```python
from build123d import *

# Parameters (mm, degrees)
SKETCH1_R           = 45
BOSS_EXTRUDE2_DEPTH = 2.5
BOSS_EXTRUDE4_START = -2.5
BOSS_EXTRUDE4_DEPTH = 2.5
CIRPATTERN1_COUNT   = 6
CUT_EXTRUDE2_DEPTH  = 2.5
SKETCH6_R           = 1.5
CUT_EXTRUDE3_DEPTH  = 5
SKETCH7_R           = 1.5875
CUT_EXTRUDE4_DEPTH  = 2.5


with BuildPart() as part:
    # Sketch1 → Boss-Extrude2 (new body)
    with BuildSketch(Plane(origin=(0, 0, 0), x_dir=(1, 0, 0), z_dir=(0, 1, 0))):
        with Locations(Location((0, 0, 0), (0, 0, 270))):
            Circle(SKETCH1_R)
    extrude(amount=BOSS_EXTRUDE2_DEPTH)

    # Sketch2 → Boss-Extrude4 (add)
    with BuildSketch(Plane(origin=(0, 2.5, 0), x_dir=(1, 0, 0), z_dir=(0, 1, 0)).offset(BOSS_EXTRUDE4_START)):
        with BuildLine():
            ThreePointArc((-42.23454554, 15.532004475), (-45, 0), (-42.23454554, -15.532004475))
            add(Edge.make_bspline(
                [(-50.212380227, -7.942360629), (-45.3159648, -11.95963121), (-42.656686571, -14.489512492), (-42.23454554, -15.532004475)],
                knots=[0.089311832, 0.089311832, 0.089311832, 0.089311832, 1, 1, 1, 1], degree=3))
            ThreePointArc((-50.212380227, -7.942360629), (-54.5, 0), (-50.212380227, 7.942360629))
            add(Edge.make_bspline(
                [(-50.212380227, 7.942360629), (-45.3159648, 11.95963121), (-42.656686571, 14.489512492), (-42.23454554, 15.532004475)],
                knots=[0.089311832, 0.089311832, 0.089311832, 0.089311832, 1, 1, 1, 1], degree=3))
        make_face()
    boss_extrude4 = extrude(amount=BOSS_EXTRUDE4_DEPTH)

    # CirPattern1: Boss-Extrude4 ×6 about axis
    cirpattern1_axis = Axis((0, 2.5, 0), (0, 1, 0))
    for i in range(1, CIRPATTERN1_COUNT):
        add(boss_extrude4.rotate(cirpattern1_axis, i * 360 / CIRPATTERN1_COUNT))

    # Sketch5 → Cut-Extrude2 (cut)
    with BuildSketch(Plane(origin=(0, 2.5, 0), x_dir=(1, 0, 0), z_dir=(0, 1, 0))):
        with BuildLine():
            Line((-8.22468756, 44.342191593), (0, 46.65782144))
            Line((0, 46.65782144), (8.22468756, 44.342191593))
            ThreePointArc((8.22468756, 44.342191593), (0, 42.851652617), (-8.22468756, 44.342191593))
        make_face()
        with BuildLine():
            Line((40.406858652, 23.32891072), (42.513808159, 15.048307431))
            ThreePointArc((42.513808159, 15.048307431), (37.11061976, 21.425826308), (34.289120599, 29.293884161))
            Line((34.289120599, 29.293884161), (40.406858652, 23.32891072))
        make_face()
        with BuildLine():
            Line((40.406858652, -23.32891072), (34.289120599, -29.293884161))
            ThreePointArc((34.289120599, -29.293884161), (37.11061976, -21.425826308), (42.513808159, -15.048307431))
            Line((42.513808159, -15.048307431), (40.406858652, -23.32891072))
        make_face()
        with BuildLine():
            Line((0, -46.65782144), (-8.22468756, -44.342191593))
            ThreePointArc((-8.22468756, -44.342191593), (0, -42.851652617), (8.22468756, -44.342191593))
            Line((8.22468756, -44.342191593), (0, -46.65782144))
        make_face()
        with BuildLine():
            Line((-40.406858652, -23.32891072), (-42.513808159, -15.048307431))
            ThreePointArc((-42.513808159, -15.048307431), (-37.11061976, -21.425826308), (-34.289120599, -29.293884161))
            Line((-34.289120599, -29.293884161), (-40.406858652, -23.32891072))
        make_face()
        with BuildLine():
            Line((-40.406858652, 23.32891072), (-34.289120599, 29.293884161))
            ThreePointArc((-34.289120599, 29.293884161), (-37.11061976, 21.425826308), (-42.513808159, 15.048307431))
            Line((-42.513808159, 15.048307431), (-40.406858652, 23.32891072))
        make_face()
    extrude(amount=-CUT_EXTRUDE2_DEPTH, mode=Mode.SUBTRACT)

    # Sketch6 → Cut-Extrude3 (cut, symmetric)
    with BuildSketch(Plane(origin=(0, 2.5, 0), x_dir=(1, 0, 0), z_dir=(0, 1, 0))):
        with Locations(Location((-45, 0, 0), (0, 0, 270))):
            Circle(SKETCH6_R)
        with Locations(Location((-22.5, 38.97114317, 0), (0, 0, 270))):
            Circle(SKETCH6_R)
        with Locations(Location((22.5, 38.97114317, 0), (0, 0, 270))):
            Circle(SKETCH6_R)
        with Locations(Location((45, 0, 0), (0, 0, 270))):
            Circle(SKETCH6_R)
        with Locations(Location((22.5, -38.97114317, 0), (0, 0, 270))):
            Circle(SKETCH6_R)
        with Locations(Location((-22.5, -38.97114317, 0), (0, 0, 270))):
            Circle(SKETCH6_R)
    extrude(amount=CUT_EXTRUDE3_DEPTH, both=True, mode=Mode.SUBTRACT)

    # Sketch7 → Cut-Extrude4 (cut)
    with BuildSketch(Plane(origin=(0, 2.5, 0), x_dir=(1, 0, 0), z_dir=(0, 1, 0))):
        with Locations(Location((-25.4, 34.29, 0), (0, 0, 270))):
            Circle(SKETCH7_R)
        with Locations(Location((-25.4, -34.29, 0), (0, 0, 270))):
            Circle(SKETCH7_R)
        with Locations(Location((25.4, -34.29, 0), (0, 0, 270))):
            Circle(SKETCH7_R)
        with Locations(Location((25.4, 34.29, 0), (0, 0, 270))):
            Circle(SKETCH7_R)
    extrude(amount=-CUT_EXTRUDE4_DEPTH, mode=Mode.SUBTRACT)


solid = part.part
```
Design review of the part built by this model. Coordinates are the model's own, in mm. Coordinates: 2 decimals unless noted, no trailing zeros. Write each loop counter-clockwise with the first axis right and the second up, starting at its lowest first coordinate (ties: lowest second). Pieces come first, ordered by that corner, then holes.
1) Mouldability with a two-part tool opening along Z and no side actions: class faces 1 (the cylindrical face through (27.364, 1.232, 47.132)), 2 (the flat face through (1, 2.5, -1)), 3 (the cylindrical face through (22.95, 1.27, -37.54)) as +Z half, -Z half, draft (parallel to the pull), parting line (faces both ways), or undercut.
2) Add section D-D (z = 25). Write out the cut boundary in (x, y), plus the area to 3 significant figures.
3) To check wall thickness, follow L1, parallel to X at y = 1.7, z = 0; L2, parallel to Z at x = -26.5, y = 1.6; L3, parallel to X at y = 0.5, z = 34.29. State the ranges of each line that lie inside material, in increasing order.
4) Add section B-B (x = -25.4). Write out the cut boundary in (y, z).
5) Insertion check: pin 1 (1.5 mm diameter, centred on y = 1.5, z = 27, fed in from +X). The pin has a flat end and moves straight along its axis. Give the tip position at first contact, or say it passes through.
6) Add section C-C (y = 0.8). State how many separate pieces and enclosed holes the cut face has, plus the area to 3 significant figures.
7) Add section A-A (z = 0). Write out the cut boundary in (x, y), plus the area to 4 significant figures.
Check result:
1. face 1: +Z half
1. face 2: draft
1. face 3: undercut
2. outline: (-35.43, 0) - (35.43, 0) - (35.43, 2.5) - (-35.43, 2.5) - close
2. area: 177 mm2
3. L1: x = -54.5 to -46.5, -43.5 to 43.5, 46.5 to 54.5
3. L2: z = -47.59 to -35.43, -33.15 to 33.15, 35.43 to 47.59
3. L3: x = -32.93 to -26.99, -23.81 to 23.81, 26.99 to 32.93
4. outline: (0, -48.02) - (2.5, -48.02) - (2.5, -35.88) - (0, -35.88) - close; (0, -32.7) - (2.5, -32.7) - (2.5, 32.7) - (0, 32.7) - close; (0, 35.88) - (2.5, 35.88) - (2.5, 48.02) - (0, 48.02) - close
5. pin 1: stops at x = 35.01
6. separate pieces: 1
6. enclosed holes: 10
6. area: 7,180 mm2
7. outline: (-54.5, 0) - (-46.5, 0) - (-46.5, 2.5) - (-54.5, 2.5) - close; (-43.5, 0) - (43.5, 0) - (43.5, 2.5) - (-43.5, 2.5) - close; (46.5, 0) - (54.5, 0) - (54.5, 2.5) - (46.5, 2.5) - close
7. area: 257.5 mm2
